```python
from build123d import *

# Parameters (mm, degrees)
BOSS_EXTRUDE2_DEPTH   = 6
M3_CLEARANCE_HOLE1_D  = 2.5
SKETCH14_R            = 3
BOSS_EXTRUDE4_DEPTH   = 6
M3_CLEARANCE_HOLE2_D  = 3.6
CIRPATTERN1_COUNT     = 6
FILLET1_R             = 6
M3X0_5_TAPPED_HOLE1_D = 3.6


with BuildPart() as part:
    # Sketch1 → Revolve1 (revolve)
    with BuildSketch(Plane.XY, mode=Mode.PRIVATE) as revolve1_sk:
        Polygon((0, 14), (6, 14), (6, 20), (14, 20), (14, 26), (0, 26), align=None)
    revolve(revolve1_sk.sketch.rotate(Axis((-2.257208118, 0, 0), (1, 0, 0)), 90), axis=Axis((-2.257208118, 0, 0), (1, 0, 0)))

    # Sketch3 → Boss-Extrude2 (add)
    with BuildSketch(Plane(origin=(0, 0, 0), x_dir=(0, 0, -1), z_dir=(1, 0, 0))):
        with BuildLine():
            ThreePointArc((24, -10), (24.831302178, -8.742992446), (26.068711806, -7.882789726))
            ThreePointArc((26.068711806, -7.882789726), (31.05103074, -5.234546759), (35.611149804, -1.911595226))
            ThreePointArc((35.611149804, -1.911595226), (36.5, 0), (35.611149804, 1.911595226))
            ThreePointArc((35.611149804, 1.911595226), (31.05103074, 5.234546759), (26.068711806, 7.882789726))
            ThreePointArc((26.068711806, 7.882789726), (24.831302178, 8.742992446), (24, 10))
            ThreePointArc((24, 10), (26, 0), (24, -10))
        make_face()
    extrude(amount=BOSS_EXTRUDE2_DEPTH)

    # M3 Clearance Hole1 (through all)
    with Locations(Plane.ZY):
        with Locations((-34, 0)):
            Hole(M3_CLEARANCE_HOLE1_D / 2)

    # Sketch14 → Boss-Extrude4 (add)
    with BuildSketch(Plane(origin=(0, 0, 0), x_dir=(0, 0, -1), z_dir=(1, 0, 0))):
        with BuildLine():
            Line((-12.5, 36.231892029), (-12.5, 22.79802623))
            ThreePointArc((-12.5, 22.79802623), (0, 26), (12.5, 22.79802623))
            Line((12.5, 22.79802623), (12.5, 36.231892029))
            ThreePointArc((12.5, 36.231892029), (11.377342361, 39.388823485), (8.513513514, 41.128093655))
            ThreePointArc((8.513513514, 41.128093655), (0, 42), (-8.513513514, 41.128093655))
            ThreePointArc((-8.513513514, 41.128093655), (-11.377342361, 39.388823485), (-12.5, 36.231892029))
        make_face()
        with Locations((0, 37)):
            Circle(SKETCH14_R, mode=Mode.SUBTRACT)
    extrude(amount=BOSS_EXTRUDE4_DEPTH)

    # M3 Clearance Hole2 (through all)
    with Locations(Plane.ZY):
        with Locations((18, 0)):
            m3_clearance_hole2 = Hole(M3_CLEARANCE_HOLE2_D / 2)

    # CirPattern1: M3 Clearance Hole2 ×6 about axis
    cirpattern1_axis = Axis((0, 0, 0), (1, 0, 0))
    for i in range(1, CIRPATTERN1_COUNT):
        add(m3_clearance_hole2.rotate(cirpattern1_axis, i * 360 / CIRPATTERN1_COUNT), mode=Mode.SUBTRACT)

    # Fillet1
    fillet1_edges = [part.edges().sort_by_distance(p)[0] for p in [
        (3, 22.79802623, 12.5),
        (3, 22.79802623, -12.5),
    ]]
    fillet(fillet1_edges, radius=FILLET1_R)

    # M3x0.5 Tapped Hole1 (through all)
    with Locations(Plane.ZY):
        with Locations((7.5, 36.231892029), (-7.5, 36.231892029)):
            Hole(M3X0_5_TAPPED_HOLE1_D / 2)


solid = part.part
```
Input: part model. Units: mm. Frame: model coordinates. A direction names the side the tool comes from. Give positions to 0.01 mm unless a question says otherwise; leave off trailing zeros. Order: outer loops, then holes, each group sorted by start corner. A loop starts at its lowest first (then second) coordinate and runs counter-clockwise, first axis right, second up.
1. Section C-C on x = 1.5. Give the number of separate pieces and of enclosed holes in the cut face, and give its area (3 significant figures).
Derived:
separate pieces: 1
enclosed holes: 11
area: 1,910 mm2
2. Section B-B on z = 17. Return the cut outline in (x, y).
Derived:
outline: (0, -19.67) - (14, -19.67) - (14, -10.54) - (6, -10.54) - (6, -1.5) - (0, -1.5) - close; (0, 1.5) - (6, 1.5) - (6, 10.54) - (14, 10.54) - (14, 19.67) - (0, 19.67) - close
3. Mould query, pull axis Y, two halves, no side actions, for faces 4 (the flat face through (6, 0, -29)), 5 (the cylindrical face through (10.06, -0.88, -19.98)), 6 (the cylindrical face through (2.96, 5.19, -31.12)). Classes: released by +Y, released by -Y, zero draft, split by the parting line, or undercut.
Derived:
face 4: zero draft
face 5: undercut
face 6: released by +Y
4. Section A-A on y = 37. Return the cut outline in (x, z).
Derived:
outline: (0, -12.44) - (6, -12.44) - (6, -9.13) - (0, -9.13) - close; (0, -5.87) - (6, -5.87) - (6, -3) - (0, -3) - close; (0, 3) - (6, 3) - (6, 5.87) - (0, 5.87) - close; (0, 9.13) - (6, 9.13) - (6, 12.44) - (0, 12.44) - close
5. Section D-D on x = 8.25. Return the cut outline in (y, z).
Derived:
outline: circle Ø52 at (0, 0); hole circle Ø40 at (0, 0)
6. Material intervals for L1, parallel to Y at x = 3.75, z = 2.5; L2, parallel to Y at x = 1.5, z = 0.5; L3, parallel to X at y = 8.5, z = 18, sorted ascending.
Derived:
L1: y = -25.88 to -13.77, 13.77 to 35.34, 38.66 to 41.93
L2: y = -26 to -13.99, 13.99 to 34.04, 39.96 to 42
L3: x = 0 to 6
7. Pin query (flat end, axial travel): pin 1 (1 mm diameter, centred on x = 10, z = -15, fed in from -Y); pin 2 (3 mm diameter, centred on x = 2.5, y = 32, fed in from -Z); pin 3 (1.5 mm diameter, centred on x = 10, y = 28.5, fed in from -Z); pin 4 (4 mm diameter, centred on y = 36.23, z = -7.5, fed in from +X). Return the tip coordinate at first contact, or that it passes through.
Derived:
pin 1: stops at y = -21.58
pin 2: stops at z = -12.5
pin 3: passes through
pin 4: stops at x = 6
8. Reachability of faces 1 (the flat face through (14, 15.3, -13.4)), 2 (the flat face through (6, -14, -4)), 3 (the flat face through (3, 31, 12.5)) from +Z, -Z, +X, -X, +Y, -Y: full face, straight path, thin tool, end or side. Return the list, or none.
Derived:
face 1: +Z, -Z, +X, +Y, -Y
face 2: +X
face 3: +Z, +X, -X, +Y
